Could you check a few things on this drawing? It's one solid part, dimensions in mm from its lowest x, y, z. Round coordinates to 2 decimals unless told otherwise and drop trailing zeros. Loops run counter-clockwise (first coordinate to the right, second up) from the corner with the lowest first, then second, coordinate; pieces in that order, holes last. Notation, with made-up numbers: (84.25, 31) -> (111.25, 31) arc R19 ccw to (111.25, 55) -> close; hole circle Ø10 at (75.5, 78). An arc over 180 degrees is marked (long way). Put each result on its own line as item: value. Start each with the question number.
1. I'm going to push flat-ended pins straight in: P1, Ø6, axis at x = 7, z = 21.5, coming from the +Y side; P2, Ø1.5, axis at x = 6, z = 11, coming from the -Y side; P3, Ø5, axis at x = 9, z = 24.5, coming from the -Y side. Where does each tip first touch, or does it pass through?
2. If we mould it in two halves opening along Z, with no side actions, what happens to the marked faces 1, 2, 3 and 4? For each: pulls with the +Z half, pulls with the -Z half, needs draft (parallel to the pull), parting line crosses it, or undercut.
3. Imagine slicing it at C-C, the plane z = 28. Please give me the cut outline in (x, y).
4. I need wall thicknesses on line 1 (Z direction, x = 8, y = 5.5); line 2 (X direction, y = 3.75, z = 6.5); line 3 (Y direction, x = 3.25, z = 15.5). Which ranges of each line are inside material? Lowest first, please. Write a range as [from, to].
5. Imagine slicing it at A-A, the plane y = 5. Please give me the cut outline in (x, z), and give its area (3 significant figures).
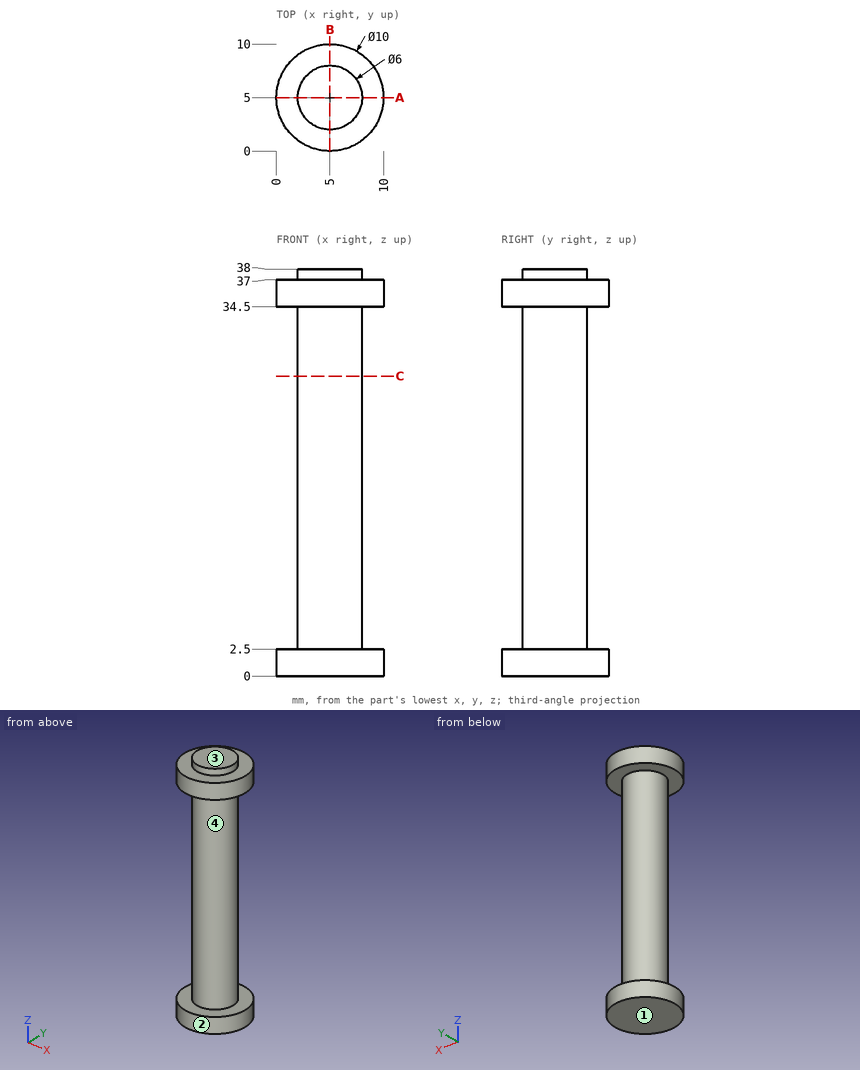
Entries:
1. P1: y = 8
1. P2: y = 2.01
1. P3: y = 2.4
2. face 1: pulls with the -Z half
2. face 2: needs draft
2. face 3: pulls with the +Z half
2. face 4: undercut
3. outline: circle Ø6 at (5, 5)
4. line 1: [0, 2.5], [34.5, 37]
4. line 2: [2.27, 7.73]
4. line 3: [2.56, 7.44]
5. outline: (0, 0) -> (10, 0) -> (10, 2.5) -> (8, 2.5) -> (8, 34.5) -> (10, 34.5) -> (10, 37) -> (8, 37) -> (8, 38) -> (2, 38) -> (2, 37) -> (0, 37) -> (0, 34.5) -> (2, 34.5) -> (2, 2.5) -> (0, 2.5) -> close
5. area: 248 mm^2
